```python
from build123d import *

# Parameters (mm, degrees)
F0_W     = 20
F0_H     = 130
F0_W_2   = 6
F0_H_2   = 13
F0_H_3   = 10
F0_W_3   = 10
F1_DEPTH = 8
F2_R     = 4
F3_DEPTH = 50
F2_W     = 20
F2_H     = 20.9063310176
F4_DEPTH = 4
F5_F1_R  = 1
F5_F2_R  = 1


with BuildPart() as f1:
    # F0 (on Top) → F1 (new body)
    with BuildSketch(Plane.XY):
        with Locations((-46.5529351234, 65.628703773)):
            Rectangle(F0_W, F0_H)
        with Locations((-46.5529351234, 8.128703773)):
            Rectangle(F0_W_2, F0_H_2, mode=Mode.SUBTRACT)
        with Locations((-46.5529351234, 34.128703773)):
            Rectangle(F0_W_2, F0_H_2, mode=Mode.SUBTRACT)
        with Locations((-46.5529351234, -4.371296227)):
            Rectangle(F0_W, F0_H_3)
        with Locations((-61.5529351234, -4.371296227)):
            Rectangle(F0_W_3, F0_H_3)
        with Locations((-31.5529351234, -4.371296227)):
            Rectangle(F0_W_3, F0_H_3)
    extrude(amount=F1_DEPTH)

    # F2 (on face) → F3 (cut, symmetric)
    with BuildSketch(Plane.XY.offset(8)):
        with Locations((-46.5529351234, 119.7651425898)):
            Circle(F2_R)
    extrude(amount=F3_DEPTH, both=True, mode=Mode.SUBTRACT)

    # F2 (on face) → F4 (join)
    with BuildSketch(Plane.XY.offset(8)):
        with Locations((-46.5529351234, 120.1755382642)):
            Rectangle(F2_W, F2_H)
        with Locations((-46.5529351234, 119.7651425898)):
            Circle(F2_R, mode=Mode.SUBTRACT)
    extrude(amount=F4_DEPTH)

    # F5: fillet of radius 1 on 35 edges, made by hand

    # F5_f1
    f5_f1_edges = [f1.edges().sort_by_distance(p)[0] for p in [
        (-46.5529351234, 109.7223727554, 8),
        (-36.5529351234, 0.628703773, 4),
        (-56.5529351234, 0.628703773, 4),
    ]]
    fillet(f5_f1_edges, radius=F5_F1_R)

    # F5_f2
    f5_f2_edges = [f1.edges().sort_by_distance(p)[0] for p in [
        (-36.5529351234, 55.1755382642, 8),
        (-31.0529351234, 0.628703773, 8),
        (-26.5529351234, -4.371296227, 8),
        (-46.5529351234, -9.371296227, 8),
        (-66.5529351234, -4.371296227, 8),
        (-62.0529351234, 0.628703773, 8),
        (-56.5529351234, 55.1755382642, 8),
        (-49.5529351234, 8.128703773, 8),
        (-46.5529351234, 1.628703773, 8),
        (-46.5529351234, 14.628703773, 8),
        (-43.5529351234, 8.128703773, 8),
        (-46.5529351234, 40.628703773, 8),
        (-49.5529351234, 34.128703773, 8),
        (-43.5529351234, 34.128703773, 8),
        (-46.5529351234, 27.628703773, 8),
        (-36.5529351234, 66.128703773, 0),
        (-56.5529351234, 66.128703773, 0),
        (-46.5529351234, 130.628703773, 12),
        (-56.5529351234, 120.1755382642, 12),
        (-46.5529351234, 109.7223727554, 12),
        (-36.5529351234, 120.1755382642, 12),
        (-50.5529351234, 119.7651425898, 12),
        (-26.5529351234, 0.628703773, 4),
        (-31.0529351234, 0.628703773, 0),
        (-66.5529351234, 0.628703773, 4),
        (-62.0529351234, 0.628703773, 0),
        (-36.5529351234, 130.628703773, 6),
        (-56.5529351234, 130.628703773, 6),
        (-46.5529351234, 130.628703773, 0),
        (-66.5529351234, -9.371296227, 4),
        (-26.5529351234, -9.371296227, 4),
        (-46.5529351234, -9.371296227, 0),
        (-56.8458283423, 0.9215969918, 0),
        (-36.2600419046, 0.9215969918, 0),
        (-56.5529351234, 109.4294795366, 8.2928932188),
        (-56.8458283423, 0.9215969918, 8),
        (-36.2600419046, 0.9215969918, 8),
        (-36.5529351234, 109.4294795366, 8.2928932188),
    ]]
    fillet(f5_f2_edges, radius=F5_F2_R)


solid = f1.part
```
Design review of the part built by this model. Coordinates are the model's own, in mm. A direction names the side the tool comes from. Round coordinates to 2 decimals unless told otherwise and drop trailing zeros. Write each loop counter-clockwise with the first axis right and the second up, starting at its lowest first coordinate (ties: lowest second). Pieces come first, ordered by that corner, then holes. Notation, with made-up numbers: (60.25, 78.25) -> (99.25, 78.25) arc R25 ccw to (99.25, 96.25) -> close; hole circle Ø8 at (57.5, 6). An arc over 180 degrees is marked (long way). Answer in a Markdown table with one row per item.
Q1. Take a section at C-C, the plane y = 65. State the section outline as (x, z) points.
The answers:
| item | result |
|---|---|
| outline | (-56.55, 1) arc R1 ccw to (-55.55, 0) -> (-37.55, 0) arc R1 ccw to (-36.55, 1) -> (-36.55, 7) arc R1 ccw to (-37.55, 8) -> (-55.55, 8) arc R1 ccw to (-56.55, 7) -> close |
Q2. Take a section at D-D, the plane x = -39.5. State the section outline as (y, z) points, then the cut area to 3 significant figures.
The answers:
| item | result |
|---|---|
| outline | (-9.37, 1) arc R1 ccw to (-8.37, 0) -> (129.63, 0) arc R1 ccw to (130.63, 1) -> (130.63, 11) arc R1 ccw to (129.63, 12) -> (110.72, 12) arc R1 ccw to (109.72, 11) -> (109.72, 9) arc R1 cw to (108.72, 8) -> (-8.37, 8) arc R1 ccw to (-9.37, 7) -> close |
| area | 1,200 mm² |
Q3. To check wall thickness, follow L1, parallel to X at y = 29, z = 5.75; L2, parallel to Y at x = -51, z = 10; L3, parallel to Y at x = -48, z = 5.25. State the ranges of each line that lie inside material, in increasing order. Write a range as [from, to].
The answers:
| item | result |
|---|---|
| L1 | [-56.55, -49.55], [-43.55, -36.55] |
| L2 | [109.72, 130.63] |
| L3 | [-9.37, 1.63], [14.63, 27.63], [40.63, 116.04], [123.49, 130.63] |
Q4. Draft analysis for pull direction X (two halves, no side actions). For faces 1 (the face through (-26.553, -4, 3)), 2 (the face through (-47.07, 123.73, 5.42)), 3 (the face through (-32, 0.629, 4)), 4 (the face through (-66.553, -4, 3)), state which applies: +X half, -X half, draft (parallel to the pull), parting line (faces both ways), or undercut.
The answers:
| item | result |
|---|---|
| face 1 | +X half |
| face 2 | undercut |
| face 3 | draft |
| face 4 | -X half |
Q5. For faces 5 (the face through (-47, 130.629, 6)), 6 (the face through (-47, 14.629, 3)), 7 (the face through (-36.553, 65, 4)), 8 (the face through (-47, 51, 8)), 9 (the face through (-62, 0.629, 4)), list the 3-axis set-ups (+Z, -Z, +X, -X, +Y, -Y) from which the entire face can be reached by the end or side of a thin tool; tool diameter is ignored.
The answers:
| item | result |
|---|---|
| face 5 | +Z, -Z, +X, -X, +Y |
| face 6 | +Z, -Z |
| face 7 | +Z, -Z, +X, +Y |
| face 8 | +Z, +X, -X, -Y |
| face 9 | +Z, -Z, -X, +Y |
Q6. Take a section at B-B, the plane x = -31. State the section outline as (y, z) points, then the cut area to 3 significant figures.
The answers:
| item | result |
|---|---|
| outline | (-9.37, 1) arc R1 ccw to (-8.37, 0) -> (-0.37, 0) arc R1 ccw to (0.63, 1) -> (0.63, 7) arc R1 ccw to (-0.37, 8) -> (-8.37, 8) arc R1 ccw to (-9.37, 7) -> close |
| area | 79.1 mm² |
Q7. Take a section at A-A, the plane y = 38.5. State the section outline as (x, z) points, then the cut area to 3 significant figures.
The answers:
| item | result |
|---|---|
| outline | (-56.55, 1) arc R1 ccw to (-55.55, 0) -> (-49.55, 0) -> (-49.55, 7) arc R1 ccw to (-50.55, 8) -> (-55.55, 8) arc R1 ccw to (-56.55, 7) -> close; (-43.55, 0) -> (-37.55, 0) arc R1 ccw to (-36.55, 1) -> (-36.55, 7) arc R1 ccw to (-37.55, 8) -> (-42.55, 8) arc R1 ccw to (-43.55, 7) -> close |
| area | 111 mm² |
Q8. Clearance check with flat-ended pins moving along their axes: pin 1 Ø2 at (y, z) = (11, 5) entering from +X; pin 2 Ø5 at (x, y) = (-46.55, 119.77) entering from +Z; pin 3 Ø6 at (x, y) = (-52.5, 47.5) entering from +Z; pin 4 Ø4 at (x, y) = (-58, 93.5) entering from -Z. State where each tip first meets the part, or that it passes through.
The answers:
| item | result |
|---|---|
| pin 1 | x = -36.55 |
| pin 2 | through |
| pin 3 | z = 8 |
| pin 4 | z = 0.11 |
